For this review, take the finished solid that the model builds, in its own axes (mm). A direction names the side the tool comes from. Round coordinates to 2 decimals unless told otherwise and drop trailing zeros. Loops run counter-clockwise (first coordinate to the right, second up) from the corner with the lowest first, then second, coordinate; pieces in that order, holes last.
1. Consider section C-C on y = -2.5. State the section outline as (x, z) points, then the cut area to 3 significant figures.
2. Draft analysis for pull direction Y (two halves, no side actions). For faces 4 (the cylindrical face through (-16.073, 3.063, 15.311)), 5 (the flat face through (5, -3, 5)), 6 (the cylindrical face through (36.469, 10.395, 15.14)), 7 (the flat face through (-21.466, -3, 15)), state which applies: released by +Y, released by -Y, zero draft, split by the parting line, or undercut.
3. Tool access review of faces 1 (the flat face through (5, -4.7, 15)), 2 (the cylindrical face through (-16.073, -8.545, 15.311)), 3 (the flat face through (31.466, -8, 12)): name each direction out of +Z, -Z, +X, -X, +Y, -Y from which nothing blocks a thin tool from reaching the whole face with its end or side.
4. Consider section B-B on x = -9. State the section outline as (y, z) points, then the cut area to 3 significant figures.
5. To check wall thickness, follow line 1 along Y through (x, z) = (-13, 21); line 2 along X through (y, z) = (-4.5, 6); line 3 along X through (y, z) = (-9.75, 15.1). State the ranges of each line that lie inside material, in increasing order.
6. Clearance check with flat-ended pins moving along their axes: pin 1 Ø1.6 at (y, z) = (-3, 19) entering from +X; pin 2 Ø5 at (y, z) = (10, 3) entering from +X; pin 3 Ø9 at (y, z) = (-9, 10.5) entering from +X; pin 4 Ø2 at (x, y) = (11, -1.5) entering from -Z. State where each tip first meets the part, or that it passes through.
Autodesk Inventor part; units mm, degrees
ref_plane "YZ Plane" through (0, 0, 0) normal (1, 0, 0) x (0, 1, 0)
ref_plane "XZ Plane" through (0, 0, 0) normal (0, 1, 0) x (-1, 0, 0)
ref_plane "XY Plane" through (0, 0, 0) normal (0, 0, 1) x (1, 0, 0)
sketch "Skizze8" plane through (0, 0, 0) normal (0, 0, 1) x (1, 0, 0)
  line L0 (-31.4655, -12.5) -> (31.4655, -12.5)
  line L1 (31.4655, -12.5) -> (31.4655, 12.5)
  line L2 (31.4655, 12.5) -> (-31.4655, 12.5)
  line L3 (-31.4655, 12.5) -> (-31.4655, -12.5)
  line L4 (-31.4655, -12.5) -> (31.4655, 12.5) construction
  line L5 (31.4655, -12.5) -> (-31.4655, 12.5) construction
  point P0 (0, 0)
  dimension "d28" = 62.931
  dimension "d29" = 25
extrude "Extrusion7" add sketch "Skizze8" along normal blind 5
sketch "Skizze9" plane through (0, 0, 5) normal (0, 0, 1) x (1, 0, 0)
  line L0 (31.4655, 12.5) -> (-31.4655, 12.5)
  line L1 (-31.4655, 12.5) -> (-31.4655, -12.5)
  line L2 (-31.4655, -12.5) -> (-21.4655, -12.5)
  line L3 (-21.4655, -12.5) -> (-21.4655, 12.5)
  line L4 (-21.4655, 12.5) -> (-31.4655, 12.5)
  line L5 (-31.4655, 12.5) -> (-31.4655, -12.5)
  point P0 (0, 0)
  dimension "d32" = 10
extrude "Extrusion8" add sketch "Skizze9" along normal blind 20
sketch "Skizze10" plane through (0, 0, 5) normal (0, 0, 1) x (1, 0, 0)
  line L0 (-21.4655, 12.5) -> (38.4655, 12.5)
  line L1 (38.4655, 12.5) -> (38.4655, -1.5)
  line L2 (38.4655, -1.5) -> (-21.4655, -1.5)
  line L3 (-21.4655, -1.5) -> (-21.4655, 12.5)
  point P0 (0, 0)
  dimension "d35" = 59.931
  dimension "d36" = 14
extrude "Extrusion9" add sketch "Skizze10" along normal blind 20
fillet "Rundung4" radius 7 2 edges at (38.4655, 12.5, 15) (38.4655, -1.5, 15)
sketch "Skizze11" plane through (0, 0, 5) normal (0, 0, 1) x (1, 0, 0)
  line L0 (31.4655, -12.5) -> (31.4655, -1.5)
  line L1 (-21.4655, -12.5) -> (31.4655, -12.5)
  line L2 (31.4655, -12.5) -> (31.4655, -4.7)
  line L3 (31.4655, -4.7) -> (-21.4655, -4.7)
  line L4 (-21.4655, -4.7) -> (-21.4655, -12.5)
  point P0 (0, 0)
  dimension "d40" = 7.8
extrude "Extrusion10" add sketch "Skizze11" along normal blind 20
sketch "Skizze12" plane through (-31.4655, -12.5, 0) normal (0, -1, 0) x (1, 0, 0)
  line L0 (0, 25) -> (62.931, 25)
  line L1 (10, 25) -> (10, 5)
  point P0 (31.4655, 0)
  point P1 (17, 15.1)
  dimension "d43" = 7
  dimension "d44" = 9.9
hole "Bohrung1" at (-14.4655, -12.5, 15.1) direction (0, 1, 0) diameter 3.242 depth 20 tip angle 118
sketch "Skizze13" plane through (0, 0, 5) normal (0, 0, -1) x (-1, 0, 0)
  arc A0 (-31.4655, 12.5) -> (-31.4655, -1.5) centre (-31.4655, 5.5) ccw
  line L0 (-31.4655, -1.5) -> (-31.4655, 12.5)
  line L1 (-31.4655, -12.5) -> (-31.4655, 12.5)
  point P0 (0, 0)
extrude "Extrusion11" add sketch "Skizze13" along normal blind 5
properties part number "Standard (DIN)"
Resolved:
1. outline: (-31.47, 0) - (31.47, 0) - (31.47, 5) - (-21.47, 5) - (-21.47, 25) - (-31.47, 25) - close
1. area: 515 mm2
2. face 4: zero draft
2. face 5: undercut
2. face 6: released by +Y
2. face 7: undercut
3. face 1: +Z, +X
3. face 2: -Y
3. face 3: +Z, -Z, +X, -Y
4. outline: (-12.5, 0) - (12.5, 0) - (12.5, 25) - (-1.5, 25) - (-1.5, 5) - (-4.7, 5) - (-4.7, 25) - (-12.5, 25) - close
4. area: 561 mm2
5. line 1: y = -12.5 to -4.7, -1.5 to 12.5
5. line 2: x = -31.47 to -21.47
5. line 3: x = -31.47 to -16.09, -12.84 to 31.47
6. pin 1: stops at x = -21.47
6. pin 2: stops at x = 38.17
6. pin 3: stops at x = 31.47
6. pin 4: stops at z = 0
